from build123d import *

# Parameters (mm, degrees)
SKETCH2_W            = 250
SKETCH2_H            = 250
BOSS_EXTRUDE1_DEPTH  = 5
SKETCH3_R            = 2
SKETCH3_R_2          = 3.05
CUT_EXTRUDE1_DEPTH   = 354.588744165
LPATTERN1_COUNT      = 2
LPATTERN1_PITCH      = 220
LPATTERN1_COUNT_DIR2 = 2
LPATTERN1_PITCH_DIR2 = 206


with BuildPart() as part:
    # Sketch2 → Boss-Extrude1 (new body)
    with BuildSketch(Plane(origin=(0, 0, 0), x_dir=(1, 0, 0), z_dir=(0, 1, 0))):
        with Locations((125, 125)):
            Rectangle(SKETCH2_W, SKETCH2_H)
    extrude(amount=BOSS_EXTRUDE1_DEPTH)

    # Sketch3 → Cut-Extrude1 (cut, through all)
    with BuildSketch(Plane(origin=(0, 5, 0), x_dir=(1, 0, 0), z_dir=(0, 1, 0))):
        with Locations(Location((22, 15, 0), (0, 0, 270))):
            Circle(SKETCH3_R)
        with Locations(Location((108.9, 134.54, 0), (0, 0, 270))):
            Circle(SKETCH3_R_2)
        with Locations(Location((127.98, 134.54, 0), (0, 0, 270))):
            Circle(SKETCH3_R_2)
        with Locations(Location((127.98, 102.34, 0), (0, 0, 270))):
            Circle(SKETCH3_R_2)
        with Locations(Location((108.9, 102.34, 0), (0, 0, 270))):
            Circle(SKETCH3_R_2)
    cut_extrude1 = extrude(amount=-CUT_EXTRUDE1_DEPTH, mode=Mode.SUBTRACT)

    # LPattern1: Cut-Extrude1 2 × 2
    with Locations(*[(j * LPATTERN1_PITCH_DIR2, 0, -i * LPATTERN1_PITCH) for i in range(LPATTERN1_COUNT) for j in range(LPATTERN1_COUNT_DIR2) if (i, j) != (0, 0)]):
        add(cut_extrude1, mode=Mode.SUBTRACT)


solid = part.part
Geometry: final body of the model. Coordinates: model frame, mm. Coordinates: 2 decimals unless noted, no trailing zeros. Order: outer loops, then holes, each group sorted by start corner. A loop starts at its lowest first (then second) coordinate and runs counter-clockwise, first axis right, second up. Notation, with made-up numbers: (80, 32.25) - (106, 32.25) arc R20 cw to (106, 41.25) - close; hole circle Ø5 at (88.5, 89.5). An arc over 180 degrees is marked (long way). Use one line per item in the form item = value.
1) Ray query, L1, parallel to Z at x = 228, y = 2.25; L2, parallel to X at y = 2.7, z = -134.54; L3, parallel to Z at x = 129, y = 1.25. Return the intervals inside material, ascending.
Solutions:
L1 = -250 to -237, -233 to -17, -13 to 0
L2 = 0 to 105.85, 111.95 to 124.93, 131.03 to 250
L3 = -250 to -137.41, -131.67 to -105.21, -99.47 to 0
2) Pin query (flat end, axial travel): pin 1 (3.5 mm diameter, centred on x = 22, z = -235, fed in from +Y). Return the tip coordinate at first contact, or that it passes through.
Solutions:
pin_1 = through
3) Mould query, pull axis X, two halves, no side actions, for faces 1 (the face through (105.923, 2.535, -135.201)), 2 (the face through (123, 0, -127)). Classes: +X half, -X half, draft (parallel to the pull), parting line (faces both ways), or undercut.
Solutions:
face_1 = undercut
face_2 = draft
4) Section B-B (z = -102.34). Return loops of the section in (x, y).
Solutions:
outline = (0, 0) - (105.85, 0) - (105.85, 5) - (0, 5) - close; (111.95, 0) - (124.93, 0) - (124.93, 5) - (111.95, 5) - close; (131.03, 0) - (250, 0) - (250, 5) - (131.03, 5) - close
5) Section A-A (x = 108.9). Return loops of the section in (y, z).
Solutions:
outline = (0, -250) - (5, -250) - (5, -137.59) - (0, -137.59) - close; (0, -131.49) - (5, -131.49) - (5, -105.39) - (0, -105.39) - close; (0, -99.29) - (5, -99.29) - (5, 0) - (0, 0) - close
